Check sheet for the modelled part. Datum: model origin and axes. Units: mm. Face numbers are marked on the shaded views. A direction names the side the tool comes from. Round coordinates to 2 decimals unless told otherwise and drop trailing zeros. Write each loop counter-clockwise with the first axis right and the second up, starting at its lowest first coordinate (ties: lowest second). Pieces come first, ordered by that corner, then holes. Notation, with made-up numbers: (38, 42.5) -> (49, 42.5) arc R17 ccw to (49, 68.5) -> close; hole circle Ø1 at (-17, 45). An arc over 180 degrees is marked (long way). Write item = value, one per line.
from build123d import *

# Parameters (mm, degrees)
BOSS_EXTRUDE1_DEPTH = 160
BOSS_EXTRUDE2_START = 60
BOSS_EXTRUDE2_DEPTH = 10
SKETCH4_W           = 2.23742312
SKETCH4_H           = 10.231207741
CUT_EXTRUDE1_DEPTH  = 175


# Read off the part's stored shape, not the designer's step: Boss-Extrude2
with BuildPart() as part:
    # Sketch1 → Boss-Extrude1 (new body)
    with BuildSketch(Plane.XY):
        Polygon((0, 0), (0, 60), (70, 60), (48.161785944, 0), align=None)
    extrude(amount=BOSS_EXTRUDE1_DEPTH)

    # Boss-Extrude2 outline → Boss-Extrude2 (add)
    with BuildSketch(Plane(origin=(0, 0, 0), x_dir=(1, 0, 0), z_dir=(0, 1, 0)).offset(BOSS_EXTRUDE2_START)):
        with BuildLine():
            ThreePointArc((45.65, -50), (30.65, -35), (15.65, -50))
            Line((15.65, -50), (15.65, -110))
            ThreePointArc((15.65, -110), (30.65, -125), (45.65, -110))
            Line((45.65, -110), (45.65, -50))
        make_face()
    extrude(amount=BOSS_EXTRUDE2_DEPTH)

    # Sketch4 → Cut-Extrude1 (cut)
    with BuildSketch(Plane.XY.offset(160)):
        with Locations((69.79871156, 58.529652548)):
            Rectangle(SKETCH4_W, SKETCH4_H)
    extrude(amount=-CUT_EXTRUDE1_DEPTH, mode=Mode.SUBTRACT)


solid = part.part
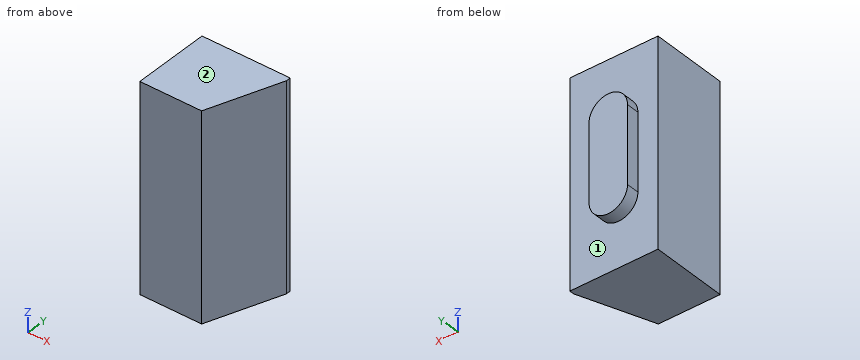
(1) Go/stop test with flat-tipped pins: P1, Ø8, axis at y = 65.5, z = 68, coming from the +X side; P2, Ø8, axis at y = 67, z = 72, coming from the -X side. Record where each tip stops, or that it passes through.
Worked answers:
P1 = 45.65
P2 = 15.65
(2) Sectioned sample at B-B on x = 30.65. Enter the section's corners in (y, z).
Worked answers:
outline = (0, 0) -> (60, 0) -> (60, 35) -> (70, 35) -> (70, 125) -> (60, 125) -> (60, 160) -> (0, 160) -> close
(3) Material ranges on L1, parallel to Y at x = 14, z = 112; L2, parallel to X at y = 22, z = 120.5; L3, parallel to X at y = 37, z = 136, recorded low to high. Write a range as [from, to].
Worked answers:
L1 = [0, 60]
L2 = [0, 56.17]
L3 = [0, 61.63]
(4) Sectioned sample at C-C on y = 24. Enter the section's corners in (x, z), then the cut area to 3 significant figures.
Worked answers:
outline = (0, 0) -> (56.9, 0) -> (56.9, 160) -> (0, 160) -> close
area = 9,100 mm²
(5) Sectioned sample at D-D on z = 17. Enter the section's corners in (x, y).
Worked answers:
outline = (0, 0) -> (48.16, 0) -> (68.68, 56.37) -> (68.68, 60) -> (0, 60) -> close
(6) Sectioned sample at A-A on z = 99. Enter the section's corners in (x, y).
Worked answers:
outline = (0, 0) -> (48.16, 0) -> (68.68, 56.37) -> (68.68, 60) -> (45.65, 60) -> (45.65, 70) -> (15.65, 70) -> (15.65, 60) -> (0, 60) -> close
(7) Access from +Z, -Z, +X, -X, +Y, -Y to the whole of each face (thin tool, end or side, straight path). Record for the marked faces 1 and 2.
Worked answers:
face_1 = +Y
face_2 = +Z, +X, -X, +Y, -Y
